```python
from build123d import *

# Parameters (mm, degrees)
F0_W     = 63.5
F0_H     = 7.9375
F0_R     = 2.38125
F1_DEPTH = 3.175
F2_DEPTH = 4.7625
F3_T     = -1.5875
F4_R     = 1.5875
F4_R_2   = 0.79375
F5_DEPTH = 1.5875


# Not quite as in the source:
# - a feature names something its author has since deleted; it is built from what else it names


with BuildPart() as f1:
    # F0 (on Top) → F1 (new body)
    with BuildSketch(Plane.XY):
        Rectangle(F0_W, F0_H)
        with Locations((-27.78125, 0)):
            Circle(F0_R, mode=Mode.SUBTRACT)
        with Locations((-19.84375, 0)):
            Circle(F0_R, mode=Mode.SUBTRACT)
        with Locations((-11.90625, 0)):
            Circle(F0_R, mode=Mode.SUBTRACT)
        with Locations((-3.96875, 0)):
            Circle(F0_R, mode=Mode.SUBTRACT)
        with Locations((3.96875, 0)):
            Circle(F0_R, mode=Mode.SUBTRACT)
        with Locations((11.90625, 0)):
            Circle(F0_R, mode=Mode.SUBTRACT)
        with Locations((19.84375, 0)):
            Circle(F0_R, mode=Mode.SUBTRACT)
        with Locations((27.78125, 0)):
            Circle(F0_R, mode=Mode.SUBTRACT)
    extrude(amount=F1_DEPTH)

    # F0 (on Top) → F2 (join)
    with BuildSketch(Plane.XY):
        with Locations((-27.78125, 0)):
            Circle(F0_R)
        with Locations((-11.90625, 0)):
            Circle(F0_R)
        with Locations((-19.84375, 0)):
            Circle(F0_R)
        with Locations((-3.96875, 0)):
            Circle(F0_R)
        with Locations((3.96875, 0)):
            Circle(F0_R)
        with Locations((11.90625, 0)):
            Circle(F0_R)
        with Locations((19.84375, 0)):
            Circle(F0_R)
        with Locations((27.78125, 0)):
            Circle(F0_R)
    extrude(amount=F2_DEPTH)

    # F3
    f3_openings = [f1.faces().sort_by_distance(p)[0] for p in [
        (0, 0, 0),
    ]]
    offset(amount=F3_T, openings=f3_openings, kind=Kind.INTERSECTION)

    # F4 (on face) → F5 (join)
    with BuildSketch(Plane(origin=(0, 0, 1.5875), x_dir=(1, 0, 0), z_dir=(0, 0, -1))):
        with Locations((-23.8125, 0)):
            Circle(F4_R)
        with Locations((-23.8125, 0)):
            Circle(F4_R_2, mode=Mode.SUBTRACT)
        with Locations((-15.875, 0)):
            Circle(F4_R)
        with Locations((-15.875, 0)):
            Circle(F4_R_2, mode=Mode.SUBTRACT)
        with Locations((-7.9375, 0)):
            Circle(F4_R)
        with Locations((-7.9375, 0)):
            Circle(F4_R_2, mode=Mode.SUBTRACT)
        Circle(F4_R)
        Circle(F4_R_2, mode=Mode.SUBTRACT)
        with Locations((7.9375, 0)):
            Circle(F4_R)
        with Locations((7.9375, 0)):
            Circle(F4_R_2, mode=Mode.SUBTRACT)
        with Locations((15.875, 0)):
            Circle(F4_R)
        with Locations((15.875, 0)):
            Circle(F4_R_2, mode=Mode.SUBTRACT)
        with Locations((23.8125, 0)):
            Circle(F4_R)
        with Locations((23.8125, 0)):
            Circle(F4_R_2, mode=Mode.SUBTRACT)
    extrude(amount=F5_DEPTH)


solid = f1.part
```
Design review of the part built by this model. Coordinates are the model's own, in mm. A direction names the side the tool comes from. Give positions to 0.01 mm unless a question says otherwise; leave off trailing zeros. Order: outer loops, then holes, each group sorted by start corner. A loop starts at its lowest first (then second) coordinate and runs counter-clockwise, first axis right, second up. Notation, with made-up numbers: (-16.75, 49.25) - (17.25, 49.25) arc R22 ccw to (17.25, 85.25) - close; hole circle Ø11 at (89, 0). An arc over 180 degrees is marked (long way). Use a Markdown table: item, result. Add a question column.
(1) Add section B-B on x = 0. Give the boundary of the cut face in (y, z) (1 decimal), then the cut area to 3 significant figures.
(2) Add section D-D on x = 12. Give the boundary of the cut face in (y, z) (1 decimal), then the cut area to 3 significant figures.
(3) Add section C-C on y = -3. Give the boundary of the cut face in (x, z) (3 decimals), then the cut area to 3 significant figures.
(4) Add section A-A on z = 0.6. Give the number of separate pieces and of enclosed holes in the cut face, then the cut area to 3 significant figures.
(5) Machinability: for faces 5 (the face through (28, 0, 3.175)), 6 (the face through (-16, -1, 0)), which of the approach directions +Z, -Z, +X, -X, +Y, -Y give a long, thin tool a straight path to every point of the face, cutting with its end or side? Answer none if there is none.
(6) Mouldability with a two-part tool opening along Y and no side actions: class faces 1 (the face through (9.527, 0.105, 3.958)), 2 (the face through (0, -3.969, 2)), 3 (the face through (-23, -1, 0)), 4 (the face through (-24, 0, 1.588)) as +Y half, -Y half, draft (parallel to the pull), parting line (faces both ways), or undercut.
(7) Wall thickness on probe 1 along Y at (x, z) = (0, 1.25); probe 2 along Z at (x, y) = (26, 1.75) (1 decimal); probe 3 along Z at (x, y) = (-7.5, 1) (3 decimals): over which ranges is each line inside the solid? List them lowest first. Write a range as [from, to].
(8) Clearance check with flat-ended pins moving along their axes: P1, Ø1.3, axis at x = 12.5, y = 0, coming from the -Z side; P2, Ø1.3, axis at x = 0, y = 0, coming from the +Z side (3 decimals); P3, Ø0.8, axis at x = 19.5, y = 0, coming from the -Z side (3 decimals). State where each tip first meets the part, or that it passes through.
Report:
| question | item | result |
|---|---|---|
| 1 | outline | (-4, 0) - (-2.4, 0) - (-2.4, 1.6) - (-1.6, 1.6) - (-1.6, 0) - (-0.8, 0) - (-0.8, 1.6) - (0.8, 1.6) - (0.8, 0) - (1.6, 0) - (1.6, 1.6) - (2.4, 1.6) - (2.4, 0) - (4, 0) - (4, 3.2) - (-4, 3.2) - close |
| 1 | area | 20.2 mm² |
| 2 | outline | (-4, 0) - (-2.4, 0) - (-2.4, 1.6) - (-0.8, 1.6) - (-0.8, 3.2) - (0.8, 3.2) - (0.8, 1.6) - (2.4, 1.6) - (2.4, 0) - (4, 0) - (4, 3.2) - (2.4, 3.2) - (2.4, 4.8) - (-2.4, 4.8) - (-2.4, 3.2) - (-4, 3.2) - close |
| 2 | area | 22.7 mm² |
| 3 | outline | (-31.75, 0) - (31.75, 0) - (31.75, 3.175) - (-31.75, 3.175) - close |
| 3 | area | 202 mm² |
| 4 | separate pieces | 8 |
| 4 | enclosed holes | 8 |
| 4 | area | 258 mm² |
| 5 | face 5 | -Z |
| 5 | face 6 | -Z, +X, -X, +Y, -Y |
| 6 | face 1 | parting line |
| 6 | face 2 | -Y half |
| 6 | face 3 | draft |
| 6 | face 4 | undercut |
| 7 | probe 1 | y = [-3.97, -2.38], [-1.59, -0.79], [0.79, 1.59], [2.38, 3.97] |
| 7 | probe 2 | z = [1.6, 3.2] |
| 7 | probe 3 | z = [0, 3.175] |
| 8 | P1 | stops at z = 1.59 |
| 8 | P2 | stops at z = 3.175 |
| 8 | P3 | stops at z = 3.175 |
